Geometry check sheet. Reference: the model listing, model coordinates, mm. A direction names the side the tool comes from. Round coordinates to 2 decimals unless told otherwise and drop trailing zeros. Write each loop counter-clockwise with the first axis right and the second up, starting at its lowest first coordinate (ties: lowest second). Pieces come first, ordered by that corner, then holes. Notation, with made-up numbers: M 43.5,66.5 L 60.5,66.5 A14 ccw 60.5,85.5 Z; hole C 31,40 d10. An arc over 180 degrees is marked long. Use a Markdown table: item, result.
```python
from build123d import *

# Parameters (mm, degrees)
SKETCH1_R           = 1.27
BOSS_EXTRUDE1_DEPTH = 2.54
SKETCH5_W           = 8.382
SKETCH5_H           = 8.382
SKETCH5_W_2         = 2.794
SKETCH5_H_2         = 43.434
CUT_EXTRUDE1_DEPTH  = 3.54
SKETCH7_R           = 1.27
CUT_EXTRUDE3_DEPTH  = 3.54
SKETCH8_W           = 12.7
SKETCH8_H           = 2.54
SKETCH8_W_2         = 2.54
SKETCH8_H_2         = 12.7
CUT_EXTRUDE4_DEPTH  = 3.54


with BuildPart() as part:
    # Sketch1 → Boss-Extrude1 (new body)
    with BuildSketch(Plane.XY):
        with BuildLine():
            Line((-3.314058103, 6.35), (48.26, 6.35))
            ThreePointArc((48.26, 6.35), (51.852102448, 4.862102448), (53.34, 1.27))
            Line((53.34, 1.27), (53.34, -92.71))
            ThreePointArc((53.34, -92.71), (51.852102448, -96.302102448), (48.26, -97.79))
            Line((48.26, -97.79), (16.846989059, -97.79))
            ThreePointArc((16.846989059, -97.79), (15.638688158, -97.644208035), (14.499741809, -97.215200367))
            Line((14.499741809, -97.215200367), (-16.7505185, -80.933552139))
            ThreePointArc((-16.7505185, -80.933552139), (-18.059258376, -79.955412607), (-18.989802686, -78.61241436))
            Line((-18.989802686, -78.61241436), (-28.309569459, -59.040904135))
            ThreePointArc((-28.309569459, -59.040904135), (-28.795802898, -57.127870198), (-28.51617555, -55.173917704))
            Line((-28.51617555, -55.173917704), (-8.107195629, 2.952923842))
            ThreePointArc((-8.107195629, 2.952923842), (-6.251501454, 5.414614163), (-3.314058103, 6.35))
        make_face()
        with Locations((48.0822, 2.286)):
            Circle(SKETCH1_R, mode=Mode.SUBTRACT)
        with Locations((-3.718687848, 1.651)):
            Circle(SKETCH1_R, mode=Mode.SUBTRACT)
        with Locations((-25.012261453, -59.761967182)):
            Circle(SKETCH1_R, mode=Mode.SUBTRACT)
    extrude(amount=BOSS_EXTRUDE1_DEPTH)

    # Sketch5 → Cut-Extrude1 (cut, through all)
    with BuildSketch(Plane(origin=(0, 0, 0), x_dir=(-1, 0, 0), z_dir=(0, 0, -1))):
        with Locations((-36.83, -17.78)):
            Rectangle(SKETCH5_W, SKETCH5_H)
        with Locations((-39.37, -45.72)):
            Rectangle(SKETCH5_W, SKETCH5_H)
        with Locations((-36.83, -27.94)):
            Rectangle(SKETCH5_W, SKETCH5_H)
        with Locations((-41.91, -64.77)):
            Rectangle(SKETCH5_W, SKETCH5_H)
        with Locations((-41.91, -83.82)):
            Rectangle(SKETCH5_W, SKETCH5_H)
        with Locations((-22.098, -17.78)):
            Rectangle(SKETCH5_W, SKETCH5_H)
        with Locations((-22.098, -27.94)):
            Rectangle(SKETCH5_W, SKETCH5_H)
        with Locations((-23.622, -45.72)):
            Rectangle(SKETCH5_W, SKETCH5_H)
        with Locations((-25.146, -64.77)):
            Rectangle(SKETCH5_W, SKETCH5_H)
        with Locations((-15.367, -26.543)):
            Rectangle(SKETCH5_W_2, SKETCH5_H_2)
        with Locations((-0.127, -26.543)):
            Rectangle(SKETCH5_W_2, SKETCH5_H_2)
    extrude(amount=-CUT_EXTRUDE1_DEPTH, mode=Mode.SUBTRACT)

    # Sketch7 → Cut-Extrude3 (cut, through all)
    with BuildSketch(Plane.XY.offset(2.54)):
        with Locations((44.2976, -2.4892)):
            Circle(SKETCH7_R)
        with Locations((18.796, -86.5378)):
            Circle(SKETCH7_R)
    extrude(amount=-CUT_EXTRUDE3_DEPTH, mode=Mode.SUBTRACT)

    # Sketch8 → Cut-Extrude4 (cut, through all)
    with BuildSketch(Plane.XY.offset(2.54)):
        with Locations((29.972, -83.312)):
            Rectangle(SKETCH8_W, SKETCH8_H)
        with Locations((20.066, -78.486)):
            Rectangle(SKETCH8_W_2, SKETCH8_H_2)
        with Locations((13.208, -81.026)):
            Rectangle(SKETCH8_W_2, SKETCH8_H_2)
        with Locations((5.588, -78.486)):
            Rectangle(SKETCH8_W_2, SKETCH8_H_2)
    extrude(amount=-CUT_EXTRUDE4_DEPTH, mode=Mode.SUBTRACT)


solid = part.part
```
Item 1: Cross-section at B-B, the plane y = -77. Record the cut outline in (x, z).
Outcome:
| item | result |
|---|---|
| outline | M -19.76,0 L 4.32,0 L 4.32,2.54 L -19.76,2.54 Z; M 6.86,0 L 11.94,0 L 11.94,2.54 L 6.86,2.54 Z; M 14.48,0 L 18.8,0 L 18.8,2.54 L 14.48,2.54 Z; M 21.34,0 L 53.34,0 L 53.34,2.54 L 21.34,2.54 Z |
Item 2: Mould release check, pull along X, two halves, no side actions. Record for faces 1 (the face through (15, -4.826, 1)), 2 (the face through (33, -97.79, 1)), 3 (the face through (-6.287, 5.389, 1.252)): +X half, -X half, draft (parallel to the pull), parting line (faces both ways), or undercut.
Outcome:
| item | result |
|---|---|
| face 1 | undercut |
| face 2 | draft |
| face 3 | -X half |
Item 3: Cross-section at C-C, the plane y = -15. Record the cut outline in (x, z).
Outcome:
| item | result |
|---|---|
| outline | M -14.41,0 L -1.27,0 L -1.27,2.54 L -14.41,2.54 Z; M 1.52,0 L 13.97,0 L 13.97,2.54 L 1.52,2.54 Z; M 16.76,0 L 17.91,0 L 17.91,2.54 L 16.76,2.54 Z; M 26.29,0 L 32.64,0 L 32.64,2.54 L 26.29,2.54 Z; M 41.02,0 L 53.34,0 L 53.34,2.54 L 41.02,2.54 Z |
Item 4: Cross-section at A-A, the plane y = -63.5. Record the cut outline in (x, z) (3 decimals).
Outcome:
| item | result |
|---|---|
| outline | M -26.186,0 L 20.955,0 L 20.955,2.54 L -26.186,2.54 Z; M 29.337,0 L 37.719,0 L 37.719,2.54 L 29.337,2.54 Z; M 46.101,0 L 53.34,0 L 53.34,2.54 L 46.101,2.54 Z |
Item 5: Go/stop test with flat-tipped pins: pin 1 (1 mm diameter, centred on x = -0.5, z = 0.5, fed in from -Y); pin 2 (1.3 mm diameter, centred on x = 15.5, z = 1.5, fed in from -Y); pin 3 (0.8 mm diameter, centred on y = -46.5, z = 1, fed in from -X); pin 4 (1.5 mm diameter, centred on x = 18.8, y = -86.54, fed in from +Z). Record where each tip stops, or that it passes through.
Outcome:
| item | result |
|---|---|
| pin 1 | stops at y = -89.66 |
| pin 2 | stops at y = -97.74 |
| pin 3 | stops at x = -25.61 |
| pin 4 | passes through |
Item 6: Material ranges on line 1 along Y through (x, z) = (34, 1); line 2 along Y through (x, z) = (22.5, 0.7); line 3 along Y through (x, z) = (25, 0.3), recorded low to high. Write a range as from..to.
Outcome:
| item | result |
|---|---|
| line 1 | y = -97.79..-84.58, -82.04..-32.13, -23.75..-21.97, -13.59..6.35 |
| line 2 | y = -97.79..-68.96, -60.58..-49.91, -41.53..-32.13, -23.75..-21.97, -13.59..6.35 |
| line 3 | y = -97.79..-84.58, -82.04..-68.96, -60.58..-49.91, -41.53..-32.13, -23.75..-21.97, -13.59..6.35 |
Item 7: Cross-section at D-D, the plane z = 1.9. Count the separate pieces of the cut face and the enclosed holes in it, and give its area (3 significant figures).
Outcome:
| item | result |
|---|---|
| separate pieces | 1 |
| enclosed holes | 20 |
| area | 6,230 mm2 |
Item 8: Access from +Z, -Z, +X, -X, +Y, -Y to the whole of each face (thin tool, end or side, straight path). Record for faces 4 (the face through (53.34, -45, 1)), 5 (the face through (21.336, -79, 1)).
Outcome:
| item | result |
|---|---|
| face 4 | +Z, -Z, +X, +Y, -Y |
| face 5 | +Z, -Z |
